from build123d import *

# Parameters (mm, degrees)
SKETCH1_R           = 1.5
BOSS_EXTRUDE1_DEPTH = 6.35


with BuildPart() as part:
    # Sketch1 → Boss-Extrude1 (new body)
    with BuildSketch(Plane(origin=(0, 0, 0), x_dir=(1, 0, 0), z_dir=(0, 1, 0))):
        with BuildLine():
            Line((0, 0), (49.85, 0))
            Line((49.85, 0), (57.85, 0))
            Line((57.85, 0), (89.35, 0))
            Line((89.35, 0), (89.35, 14.83))
            ThreePointArc((89.35, 14.83), (54.779581991, 78), (89.35, 141.17))
            Line((89.35, 141.17), (89.35, 156))
            Line((89.35, 156), (57.85, 156))
            Line((57.85, 156), (49.85, 156))
            Line((49.85, 156), (0, 156))
            Line((0, 156), (0, 124.7))
            Line((0, 124.7), (0, 31.3))
            Line((0, 31.3), (0, 0))
        make_face()
        with Locations(Location((45, 26.3, 0), (0, 0, 270))):
            Circle(SKETCH1_R, mode=Mode.SUBTRACT)
        with Locations(Location((45, 4.3, 0), (0, 0, 270))):
            Circle(SKETCH1_R, mode=Mode.SUBTRACT)
        with Locations(Location((15, 26.3, 0), (0, 0, 270))):
            Circle(SKETCH1_R, mode=Mode.SUBTRACT)
        with Locations(Location((5, 26.3, 0), (0, 0, 270))):
            Circle(SKETCH1_R, mode=Mode.SUBTRACT)
        with Locations(Location((53.85, 26.3, 0), (0, 0, 270))):
            Circle(SKETCH1_R, mode=Mode.SUBTRACT)
        with Locations(Location((53.85, 4.3, 0), (0, 0, 270))):
            Circle(SKETCH1_R, mode=Mode.SUBTRACT)
        with Locations(Location((53.85, 151.7, 0), (0, 0, 90))):
            Circle(SKETCH1_R, mode=Mode.SUBTRACT)
        with Locations(Location((53.85, 129.7, 0), (0, 0, 90))):
            Circle(SKETCH1_R, mode=Mode.SUBTRACT)
        with Locations(Location((5, 129.7, 0), (0, 0, 90))):
            Circle(SKETCH1_R, mode=Mode.SUBTRACT)
        with Locations(Location((15, 129.7, 0), (0, 0, 90))):
            Circle(SKETCH1_R, mode=Mode.SUBTRACT)
        with Locations(Location((45, 151.7, 0), (0, 0, 90))):
            Circle(SKETCH1_R, mode=Mode.SUBTRACT)
        with Locations(Location((45, 129.7, 0), (0, 0, 90))):
            Circle(SKETCH1_R, mode=Mode.SUBTRACT)
        with Locations(Location((5, 118, 0), (0, 0, 270))):
            Circle(SKETCH1_R, mode=Mode.SUBTRACT)
        with Locations(Location((5, 78, 0), (0, 0, 270))):
            Circle(SKETCH1_R, mode=Mode.SUBTRACT)
        with Locations(Location((5, 38, 0), (0, 0, 90))):
            Circle(SKETCH1_R, mode=Mode.SUBTRACT)
        with Locations(Location((12.62, 38, 0), (0, 0, 90))):
            Circle(SKETCH1_R, mode=Mode.SUBTRACT)
        with Locations(Location((12.62, 78, 0), (0, 0, 270))):
            Circle(SKETCH1_R, mode=Mode.SUBTRACT)
        with Locations(Location((12.62, 118, 0), (0, 0, 270))):
            Circle(SKETCH1_R, mode=Mode.SUBTRACT)
        with Locations(Location((20.24, 38, 0), (0, 0, 90))):
            Circle(SKETCH1_R, mode=Mode.SUBTRACT)
        with Locations(Location((20.24, 78, 0), (0, 0, 270))):
            Circle(SKETCH1_R, mode=Mode.SUBTRACT)
        with Locations(Location((20.24, 118, 0), (0, 0, 270))):
            Circle(SKETCH1_R, mode=Mode.SUBTRACT)
    extrude(amount=BOSS_EXTRUDE1_DEPTH)


solid = part.part
Here's how the part is built. I have some questions about the finished solid (model axes, mm). Coordinates: 2 decimals unless noted, no trailing zeros. Write each loop counter-clockwise with the first axis right and the second up, starting at its lowest first coordinate (ties: lowest second). Pieces come first, ordered by that corner, then holes.
Item 1: I want a section at B-B on x = 45. Write out the boundary of the cut face in (y, z), and give its area (3 significant figures).
Item 2: If we mould it in two halves opening along X, with no side actions, what happens to faces 1 (the cylindrical face through (5.07, 3.13, -119.5)), 2 (the flat face through (34, 0, -79))? For each: +X half, -X half, draft (parallel to the pull), parting line (faces both ways), or undercut.
Item 3: I want a section at A-A on z = -151.7. Write out the boundary of the cut face in (x, y), and give its area (3 significant figures).
Item 4: I want a section at C-C on y = 2. Count the separate pieces of the cut face and the enclosed holes in it, and give its area (3 significant figures).
Item 5: If I drill on line 1 (X direction, y = 2.75, z = -78); line 2 (X direction, y = 1.5, z = -151.7); line 3 (Z direction, x = 13, y = 6), over which ranges is the centre line in solid material (lowest first)?
Item 6: Will this pin go through, and if not, where does the flat tip stop? pin 1 (2 mm diameter, centred on x = 16.5, z = -28.5, fed in from -Y).
Item 7: I want a section at D-D on x = 5. Write out the boundary of the cut face in (y, z).
Findings below:
1. outline: (0, -156) - (6.35, -156) - (6.35, -153.2) - (0, -153.2) - close; (0, -150.2) - (6.35, -150.2) - (6.35, -131.2) - (0, -131.2) - close; (0, -128.2) - (6.35, -128.2) - (6.35, -27.8) - (0, -27.8) - close; (0, -24.8) - (6.35, -24.8) - (6.35, -5.8) - (0, -5.8) - close; (0, -2.8) - (6.35, -2.8) - (6.35, 0) - (0, 0) - close
1. area: 914 mm2
2. face 1: undercut
2. face 2: draft
3. outline: (0, 0) - (43.5, 0) - (43.5, 6.35) - (0, 6.35) - close; (46.5, 0) - (52.35, 0) - (52.35, 6.35) - (46.5, 6.35) - close; (55.35, 0) - (89.35, 0) - (89.35, 6.35) - (55.35, 6.35) - close
3. area: 529 mm2
4. separate pieces: 1
4. enclosed holes: 21
4. area: 10,700 mm2
5. line 1: x = 0 to 3.5, 6.5 to 11.12, 14.12 to 18.74, 21.74 to 54.78
5. line 2: x = 0 to 43.5, 46.5 to 52.35, 55.35 to 89.35
5. line 3: z = -156 to -119.45, -116.55 to -79.45, -76.55 to -39.45, -36.55 to 0
6. pin 1: stops at y = 0
7. outline: (0, -156) - (6.35, -156) - (6.35, -131.2) - (0, -131.2) - close; (0, -128.2) - (6.35, -128.2) - (6.35, -119.5) - (0, -119.5) - close; (0, -116.5) - (6.35, -116.5) - (6.35, -79.5) - (0, -79.5) - close; (0, -76.5) - (6.35, -76.5) - (6.35, -39.5) - (0, -39.5) - close; (0, -36.5) - (6.35, -36.5) - (6.35, -27.8) - (0, -27.8) - close; (0, -24.8) - (6.35, -24.8) - (6.35, 0) - (0, 0) - close
